Read the model definition and answer for the solid it produces. Units are mm, in the model's axes. Give positions to 0.01 mm unless a question says otherwise; leave off trailing zeros. Loops run counter-clockwise (first coordinate to the right, second up) from the corner with the lowest first, then second, coordinate; pieces in that order, holes last. Notation, with made-up numbers: (11, 79.25) - (31, 79.25) arc R28 ccw to (31, 118.25) - close; hole circle Ø3 at (49, 35.5). An arc over 180 degrees is marked (long way). Write item = value, one per line. Start each with the question number.
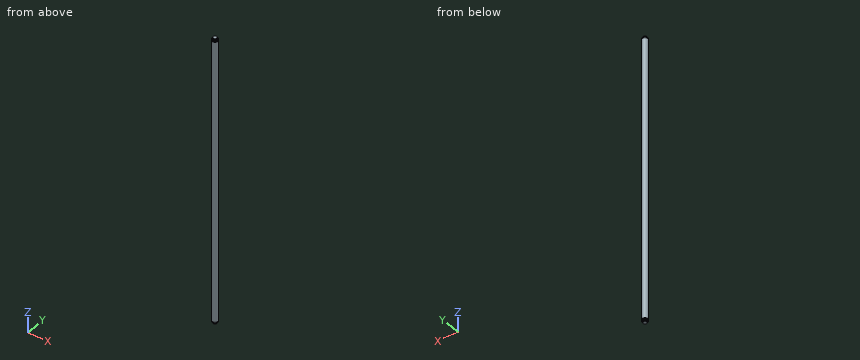
from build123d import *


with BuildPart() as part:
    # Esboço2 → Revolução1 (revolve)
    with BuildSketch(Plane(origin=(0, 0, 0), x_dir=(1, 0, 0), z_dir=(0, 1, 0)), mode=Mode.PRIVATE) as revolu_o1_sk:
        Polygon((-2.5, 0), (0, 0), (0, 400), (-2.5, 400), (-3.1, 399.4), (-3.1, 398.8), (-2.6, 398.8), (-2.6, 398), (-3.5, 398), (-4, 397.5), (-4, 397), (-3.5, 397), (-3.5, 396.2), (-4, 396.2), (-4, 3.8), (-3.5, 3.8), (-3.5, 3), (-4, 3), (-4, 2.5), (-3.5, 2), (-2.6, 2), (-2.6, 1.2), (-3.1, 1.2), (-3.1, 0.6), align=None)
    revolve(revolu_o1_sk.sketch.rotate(Axis((0, 0, 0), (0, 0, -1)), 180), axis=Axis((0, 0, 0), (0, 0, -1)))


solid = part.part
1. A cutting plane is placed at A-A on z = -355.5. Give the vertices of the cut face in (x, y), and give its area (3 significant figures).
2. Given P1, Ø2, axis at x = -2.5, z = -244.5, coming from the -Y side; P2, Ø1, axis at x = -1, y = 0.5, coming from the +Z side, each flat-ended and moving along its own axis, determine where each tip first touches the part or whether it passes through.
3. Consider line 1 along Y through (x, z) = (-0.75, -172.5); line 2 along X through (y, z) = (-0.25, -196); line 3 along Z through (x, y) = (1.5, -2.75). Determine where each line is inside the solid, lowest interval first. Write a range as [from, to].
Reply:
q1.outline = circle Ø8 at (0, 0)
q1.area = 50.3 mm^2
q2.P1 = -3.71
q2.P2 = 0
q3.line_1 = [-3.93, 3.93]
q3.line_2 = [-3.99, 3.99]
q3.line_3 = [-398, -2]
